```python
from build123d import *

# Parameters (mm, degrees)
F0_W      = 250
F0_H      = 50
F1_DEPTH  = 20
F2_W      = 10.137797147
F2_H      = 50
F3_DEPTH  = 55
F5_DEPTH  = 200.001
F6_W      = 12.0579496026
F6_H      = 50
F7_DEPTH  = 55
F9_DEPTH  = 12.0579496026
F10_DEPTH = 2


with BuildPart() as f1:
    # F0 (on Top) → F1 (new body)
    with BuildSketch(Plane.XY):
        with Locations((2.2913627326, -47.1521499132)):
            Rectangle(F0_W, F0_H)
    extrude(amount=F1_DEPTH)

    # F2 (on face) → F3 (join)
    with BuildSketch(Plane.XY.offset(20)):
        with Locations((72.2224641591, -47.1521499132)):
            Rectangle(F2_W, F2_H)
    extrude(amount=F3_DEPTH)

    # F4 (on face) → F5 (cut, through all)
    with BuildSketch(Plane.YZ.offset(77.2913627326)):
        with BuildLine():
            ThreePointArc((-63.6521499132, 75), (-47.1521499132, 58.5), (-30.6521499132, 75))
            Line((-30.6521499132, 75), (-63.6521499132, 75))
        make_face()
    extrude(amount=-F5_DEPTH, mode=Mode.SUBTRACT)

    # F6 (on face) → F7 (join, through all)
    with BuildSketch(Plane.XY.offset(20)):
        with Locations((-66.679662466, -47.1521499132)):
            Rectangle(F6_W, F6_H)
    extrude(amount=F7_DEPTH)

    # F8 (on face) → F9 (cut, through all)
    with BuildSketch(Plane(origin=(-72.7086372674, 0, 0), x_dir=(0, -1, 0), z_dir=(-1, 0, 0))):
        with BuildLine():
            ThreePointArc((25.6521499132, 75), (47.1521499132, 53.5), (68.6521499132, 75))
            Line((68.6521499132, 75), (25.6521499132, 75))
        make_face()
    extrude(amount=-F9_DEPTH, mode=Mode.SUBTRACT)

    # F10 (cut): a face of the model
    f10_faces = [f1.faces().sort_by_distance(p)[0] for p in [
        (-60.6506876647, -47.1521499132, 40.9076845732),
    ]]
    extrude(f10_faces, amount=-F10_DEPTH, mode=Mode.SUBTRACT)


solid = f1.part
```
Can you work these out from the model? Positions are in its coordinate system, mm. A direction names the side the tool comes from. Coordinates: 2 decimals unless noted, no trailing zeros. Loops run counter-clockwise (first coordinate to the right, second up) from the corner with the lowest first, then second, coordinate; pieces in that order, holes last. Notation, with made-up numbers: (17.5, -31.5) -> (34.5, -31.5) arc R6 cw to (34.5, -20.5) -> close; hole circle Ø7 at (58.5, 9). An arc over 180 degrees is marked (long way). Answer as a JSON object with one key per item and string values.
1) For faces 5 (the face through (77.291, -48, 41)), 6 (the face through (1, -47, 20)), 7 (the face through (-67.75, -46.679, 53.505)), 8 (the face through (-72.709, -48, 41)), which set-ups out of +Z, -Z, +X, -X, +Y, -Y let a thin tool reach every point of the face, with its end or its side?
Results:
{"face 5": "+Z, +X, +Y, -Y", "face 6": "+Z, +Y, -Y", "face 7": "+Z, -X", "face 8": "+Z, -X, +Y, -Y"}
2) Imagine slicing it at A-A (z = 26.5). Please give me the cut outline in (x, y).
Results:
{"outline": "(-72.71, -72.15) -> (-62.65, -72.15) -> (-62.65, -22.15) -> (-72.71, -22.15) -> close; (67.15, -72.15) -> (77.29, -72.15) -> (77.29, -22.15) -> (67.15, -22.15) -> close"}
3) For P1, Ø15, axis at y = -46, z = 54.5, coming from the -X side; P2, Ø25, axis at x = -103.5, y = -47, coming from the +Z side; P3, Ø15, axis at y = -52, z = 50.5, coming from the +X side, each with a flat end and sliding along its axis, tell me the tip position at first contact or that it passes through.
Results:
{"P1": "stops at x = -72.71", "P2": "stops at z = 20", "P3": "stops at x = 77.29"}
4) Thinking about a two-plate mould opening in Y: for faces 1 (the face through (-8, -22.152, 15)), 2 (the face through (-98, -47, 20)), 3 (the face through (72.293, -47.515, 58.504)), 4 (the face through (-8, -72.152, 15)), which applies, pulls with the +Y half, pulls with the -Y half, needs draft (parallel to the pull), parting line crosses it, or undercut?
Results:
{"face 1": "pulls with the +Y half", "face 2": "needs draft", "face 3": "undercut", "face 4": "pulls with the -Y half"}
5) Imagine slicing it at B-B (y = -59.5). Please give me the cut outline in (x, z).
Results:
{"outline": "(-122.71, 0) -> (127.29, 0) -> (127.29, 20) -> (77.29, 20) -> (77.29, 64.06) -> (67.15, 64.06) -> (67.15, 20) -> (-62.65, 20) -> (-62.65, 57.4) -> (-72.71, 57.4) -> (-72.71, 20) -> (-122.71, 20) -> close"}
6) If I drill on line 1 (X direction, y = -41.5, z = 41.5); line 2 (Z direction, x = -93, y = -64); line 3 (X direction, y = -62, z = 67), over which ranges is the centre line in solid material (lowest first)?
Results:
{"line 1": "x = -72.71 to -62.65, 67.15 to 77.29", "line 2": "z = 0 to 20", "line 3": "x = 67.15 to 77.29"}
7) Imagine slicing it at C-C (z = 70). Please give me the cut outline in (x, y).
Results:
{"outline": "(-72.71, -72.15) -> (-62.65, -72.15) -> (-62.65, -68.06) -> (-72.71, -68.06) -> close; (-72.71, -26.24) -> (-62.65, -26.24) -> (-62.65, -22.15) -> (-72.71, -22.15) -> close; (67.15, -72.15) -> (77.29, -72.15) -> (77.29, -62.88) -> (67.15, -62.88) -> close; (67.15, -31.43) -> (77.29, -31.43) -> (77.29, -22.15) -> (67.15, -22.15) -> close"}
8) Imagine slicing it at D-D (x = -80.5). Please give me the cut outline in (y, z).
Results:
{"outline": "(-72.15, 0) -> (-22.15, 0) -> (-22.15, 20) -> (-72.15, 20) -> close"}
